Drawing for the job (mm, zero at the part's lowest x, y, z). Round coordinates to 2 decimals unless told otherwise and drop trailing zeros. Order: outer loops, then holes, each group sorted by start corner. A loop starts at its lowest first (then second) coordinate and runs counter-clockwise, first axis right, second up. Notation, with made-up numbers: M -23,19.5 L -9,19.5 A26 cw -9,52.5 Z; hole C 79,-30 d4. An arc over 180 degrees is marked long. Answer as CSV lines item,"result". Start each with the question number.
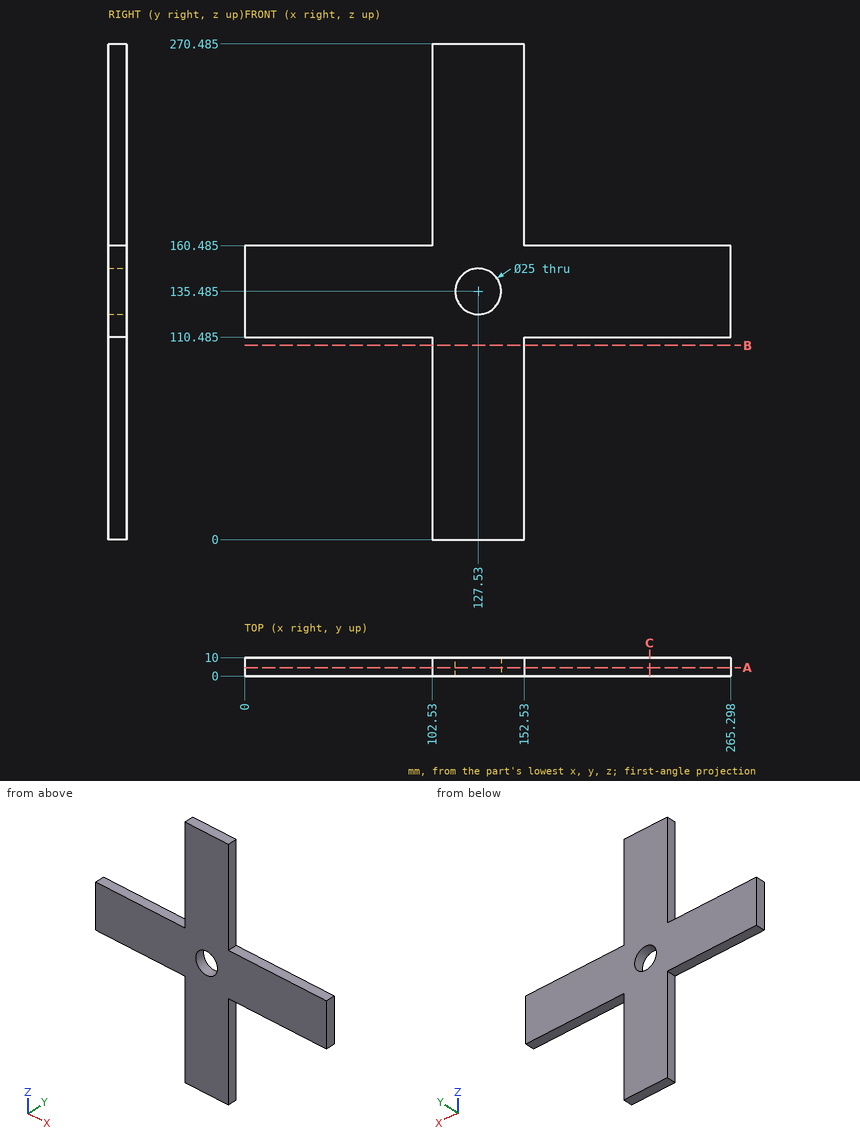
Q1. Drop flat-ended pins along their axis: P1, Ø3, axis at x = 53, y = 5.5, coming from the -Z side (1 decimal); P2, Ø3, axis at y = 6, z = 66.5, coming from the +X side; P3, Ø6, axis at x = 173, y = 5.5, coming from the +Z side (1 decimal). Give the stop position or say it passes through.
Q2. Band-saw the part on C-C, the plane x = 221. Write the cut outline in (y, z) (1 decimal).
Q3. Probe line 1 along Z through (x, y) = (156, 7.25) (1 decimal); line 2 along X through (y, z) = (9.25, 102); line 3 along X through (y, z) = (5.75, 142). List the from-to ranges inside material, lowest first. Write a range as from..to.
Q4. Band-saw the part on B-B, the plane z = 106. Write the cut outline in (x, y), then the cut area to 3 significant figures.
Q5. Band-saw the part on A-A, the plane y = 4.5. Write the cut outline in (x, z) (1 decimal), then the cut area to 3 significant figures.
Answer:
1,P1,"stops at z = 110.5"
1,P2,"stops at x = 152.53"
1,P3,"stops at z = 160.5"
2,outline,"M 0,110.5 L 10,110.5 L 10,160.5 L 0,160.5 Z"
3,line 1,"z = 110.5..160.5"
3,line 2,"x = 102.53..152.53"
3,line 3,"x = 0..116.86, 138.2..265.3"
4,outline,"M 102.53,0 L 152.53,0 L 152.53,10 L 102.53,10 Z"
4,area,"500 mm^2"
5,outline,"M 0,110.5 L 102.5,110.5 L 102.5,0 L 152.5,0 L 152.5,110.5 L 265.3,110.5 L 265.3,160.5 L 152.5,160.5 L 152.5,270.5 L 102.5,270.5 L 102.5,160.5 L 0,160.5 Z; hole C 127.5,135.5 d25"
5,area,"23,800 mm^2"
